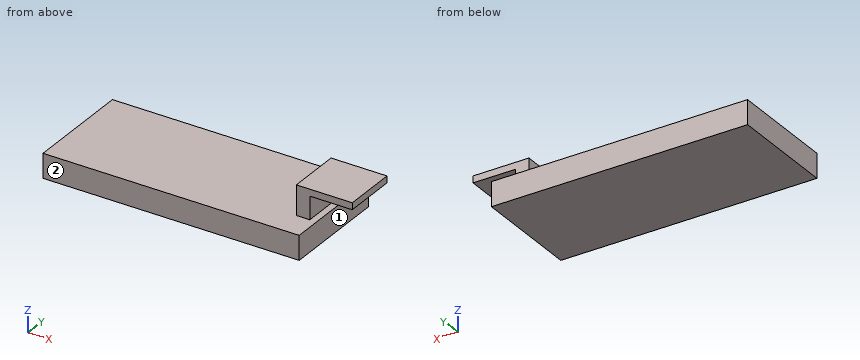
from build123d import *

# Parameters (mm, degrees)
F0_W     = 38
F0_H     = 16
F1_DEPTH = 3.6
F4_DEPTH = 3.4
F7_DEPTH = 1


with BuildPart() as f1:
    # F0 (on Top) → F1 (new body)
    with BuildSketch(Plane.XY):
        with Locations((19, -8)):
            Rectangle(F0_W, F0_H)
    extrude(amount=F1_DEPTH)

    # F3 (on offset) → F4 (join)
    with BuildSketch(Plane.XY.offset(3.6)):
        Polygon((37, -4), (35, -4), (35, -12), (37, -12), (37, -8), align=None)
    extrude(amount=F4_DEPTH)

    # F6 (on offset) → F7 (join)
    with BuildSketch(Plane.XY.offset(7)):
        Polygon((43.3, -12), (43.3, -8), (43.3, -4), (35, -4), (35, -12), align=None)
    extrude(amount=F7_DEPTH)


solid = f1.part
Source: CAD feature listing. Evaluate the final solid. Frame: model axes, mm. Face numbers are marked on the shaded views. A direction names the side the tool comes from. Round coordinates to 2 decimals unless told otherwise and drop trailing zeros. Loops run counter-clockwise (first coordinate to the right, second up) from the corner with the lowest first, then second, coordinate; pieces in that order, holes last.
Q1. Access query for the marked faces 1 and 2. Directions: +Z, -Z, +X, -X, +Y, -Y. A direction counts if a zero-diameter tool reaches every point of the face in a straight line with its end or side. Return the directions, or none.
Q2. Section B-B, the plane z = 2.25. Return loops of the section in (x, y).
Q3. Section A-A, the plane y = -5. Return loops of the section in (x, z), plus the area to 3 significant figures.
Q4. Section C-C, the plane x = 21. Return loops of the section in (y, z), plus the area to 3 significant figures.
Q5. First-contact query: P1, Ø1.3, axis at x = 40.5, z = 5, coming from the -Y side; P2, Ø8, axis at x = 19.5, y = -11, coming from the +Z side; P3, Ø3.5, axis at x = 38, z = 6, coming from the +Y side; P4, Ø2, axis at y = -6.5, z = 5, coming from the +X side. Flat tips, straight axial feed; report the tip coordinate or a pass-through.
Q6. Ray query, line 1 (Z direction, x = 37.5, y = -6.5); line 2 (X direction, y = -14.5, z = 1); line 3 (Z direction, x = 22, y = -11.75). Return the intervals inside material, ascending.
Solutions:
1. face 1: -Z, +X, +Y, -Y
1. face 2: +Z, -Z, +X, -X, -Y
2. outline: (0, -16) - (38, -16) - (38, 0) - (0, 0) - close
3. outline: (0, 0) - (38, 0) - (38, 3.6) - (37, 3.6) - (37, 7) - (43.3, 7) - (43.3, 8) - (35, 8) - (35, 3.6) - (0, 3.6) - close
3. area: 152 mm2
4. outline: (-16, 0) - (0, 0) - (0, 3.6) - (-16, 3.6) - close
4. area: 57.6 mm2
5. P1: passes through
5. P2: stops at z = 3.6
5. P3: stops at y = -4
5. P4: stops at x = 37
6. line 1: z = 0 to 3.6, 7 to 8
6. line 2: x = 0 to 38
6. line 3: z = 0 to 3.6
